from build123d import *

# Parameters (mm, degrees)
SKETCH5_R           = 3.175
BOSS_EXTRUDE3_DEPTH = 63.5
CHAMFER1_SIZE       = 0.9525
BOSS_EXTRUDE4_DEPTH = 3.96875
SKETCH8_OUTSIDE_W   = 264.208
SKETCH8_OUTSIDE_H   = 265.928
SKETCH8_OUTSIDE_R   = 5.55625
CUT_EXTRUDE3_DEPTH  = 68.46875
CUT_EXTRUDE3_TAPER  = 60
CUT_EXTRUDE4_DEPTH  = 0.254
CIRPATTERN1_COUNT   = 3


with BuildPart() as part:
    # Sketch5 → Boss-Extrude3 (new body)
    with BuildSketch(Plane(origin=(33.734375, 0, 0), x_dir=(0, 0, -1), z_dir=(1, 0, 0))):
        Circle(SKETCH5_R)
    extrude(amount=-BOSS_EXTRUDE3_DEPTH)

    # Chamfer1
    chamfer1_edges = [part.edges().sort_by_distance(p)[0] for p in [
        (33.734375, 0, 3.175),
    ]]
    chamfer(chamfer1_edges, length=CHAMFER1_SIZE)

    # Sketch11 → Revolve1 (revolve)
    with BuildSketch(Plane.XY):
        Polygon((-29.765625, 3.175), (-29.765625, 0), (17.859375, 0), (14.684375, 3.175), align=None)
    revolve(axis=Axis((-29.765625, 0, 0), (1, 0, 0)))

    # Sketch6 → Boss-Extrude4 (add)
    with BuildSketch(Plane.ZY.offset(29.765625)):
        Polygon((5.55625, 3.207902433), (0, 6.415804866), (-5.55625, 3.207902433), (-5.55625, -3.207902433), (0, -6.415804866), (5.55625, -3.207902433), align=None)
    extrude(amount=BOSS_EXTRUDE4_DEPTH)

    # Sketch8 outside → Cut-Extrude3 (cut, through all)
    with BuildSketch(Plane.ZY.offset(33.734375)):
        Rectangle(SKETCH8_OUTSIDE_W, SKETCH8_OUTSIDE_H)
        Circle(SKETCH8_OUTSIDE_R, mode=Mode.SUBTRACT)
    extrude(amount=-CUT_EXTRUDE3_DEPTH, taper=CUT_EXTRUDE3_TAPER, mode=Mode.SUBTRACT)

    # Sketch12 → Cut-Extrude4 (cut)
    with BuildSketch(Plane.ZY.offset(33.734375)):
        with BuildLine():
            Line((0.1666875, 4.2783125), (0.1666875, 2.3891875))
            ThreePointArc((0.1666875, 2.3891875), (0, 2.2225), (-0.1666875, 2.3891875))
            Line((-0.1666875, 2.3891875), (-0.1666875, 4.2783125))
            ThreePointArc((-0.1666875, 4.2783125), (0, 4.445), (0.1666875, 4.2783125))
        make_face()
    cut_extrude4 = extrude(amount=-CUT_EXTRUDE4_DEPTH, mode=Mode.SUBTRACT)

    # CirPattern1: Cut-Extrude4 ×3 about axis
    cirpattern1_axis = Axis((0, 0, 0), (1, 0, 0))
    for i in range(1, CIRPATTERN1_COUNT):
        add(cut_extrude4.rotate(cirpattern1_axis, i * 360 / CIRPATTERN1_COUNT), mode=Mode.SUBTRACT)


solid = part.part
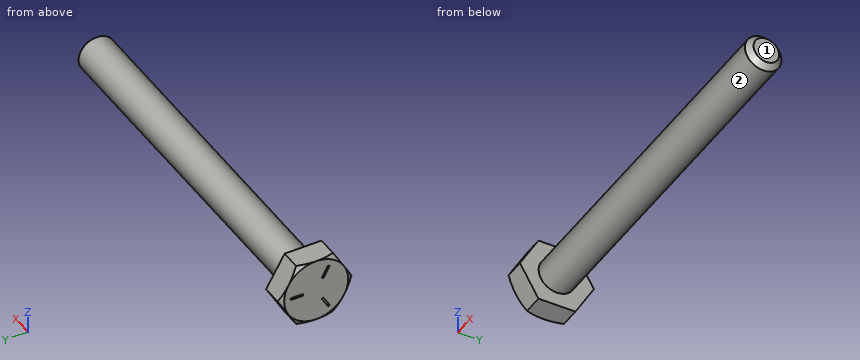
Read the model definition and answer for the solid it produces. Units are mm, in the model's axes. Face numbers are marked on the shaded views. A direction names the side the tool comes from. Round coordinates to 2 decimals unless told otherwise and drop trailing zeros. Loops run counter-clockwise (first coordinate to the right, second up) from the corner with the lowest first, then second, coordinate; pieces in that order, holes last. Notation, with made-up numbers: (52, 50) - (84, 50) arc R29 ccw to (84, 80) - close; hole circle Ø10 at (81.5, 23). An arc over 180 degrees is marked (long way). One line per question, with ' | ' between items. Start each with the question number.
Q1. Section A-A on x = 10 is taken. Give the vertices of the cut face in (y, z) (3 decimals).
Q2. For the marked faces 1 and 2, determine the directions among +Z, -Z, +X, -X, +Y, -Y from which every point of the face is accessible in a straight line to the end or side of a thin tool.
Q3. Find the intervals of material crossed by L1, parallel to X at y = 2.75, z = -4.25; L2, parallel to Z at x = -0.5, y = 0 (3 decimals), in increasing order.
Q4. Flat-ended cylindrical pins translate along their axes: pin 1 (4 mm diameter, centred on x = -4, y = -1.5, fed in from -Z) (3 decimals); pin 2 (4 mm diameter, centred on x = -7, z = 4, fed in from +Y); pin 3 (2 mm diameter, centred on x = -5, y = 5, fed in from +Z); pin 4 (2 mm diameter, centred on x = -14, y = -3, fed in from +Z). Find the tip coordinate at first contact, or state that the pin passes through.
Established:
1) outline: circle Ø6.35 at (0, 0)
2) face 1: +Z, -Z, +X, +Y, -Y | face 2: +X
3) L1: -33.73 to -29.77 | L2: -3.175 to 3.175
4) pin 1: z = -3.175 | pin 2: y = 2.47 | pin 3: through | pin 4: z = 2.47
